```python
from build123d import *

# Parameters (mm, degrees)
CHAMFER1_SIZE      = 0.8
CHAMFER2_SIZE      = 0.5
CUT_EXTRUDE1_DEPTH = 2.5
CHAMFER3_SIZE      = 0.4


with BuildPart() as part:
    # Sketch1 → Revolve1 (revolve)
    with BuildSketch(Plane.XY):
        Polygon((0, 0), (0, 4.25), (5, 4.25), (5, 2.488), (55, 2.488), (55, 0), align=None)
    revolve(axis=Axis((-88.705490849, 0, 0), (1, 0, 0)))

    # Chamfer1
    chamfer1_edges = [part.edges().sort_by_distance(p)[0] for p in [
        (55, -2.488, 0),
    ]]
    chamfer(chamfer1_edges, length=CHAMFER1_SIZE)

    # Chamfer2
    chamfer2_edges = [part.edges().sort_by_distance(p)[0] for p in [
        (0, -4.25, 0),
    ]]
    chamfer(chamfer2_edges, length=CHAMFER2_SIZE)

    # Sketch3 → Cut-Extrude1 (cut)
    with BuildSketch(Plane(origin=(0, 0, 0), x_dir=(0, 0, -1), z_dir=(1, 0, 0))):
        Polygon((-2.309401077, 0), (-1.154700538, -2), (1.154700538, -2), (2.309401077, 0), (1.154700538, 2), (-1.154700538, 2), align=None)
    extrude(amount=CUT_EXTRUDE1_DEPTH, mode=Mode.SUBTRACT)

    # Chamfer3
    chamfer3_edges = [part.edges().sort_by_distance(p)[0] for p in [
        (0, 1, 1.732050808),
        (0, -1, 1.732050808),
        (0, -2, 0),
        (0, -1, -1.732050808),
        (0, 1, -1.732050808),
        (0, 2, 0),
    ]]
    chamfer(chamfer3_edges, length=CHAMFER3_SIZE)


solid = part.part
```
Build history of the part. All positions in model axes, mm. A direction names the side the tool comes from. Give positions to 0.01 mm unless a question says otherwise; leave off trailing zeros. Loops run counter-clockwise (first coordinate to the right, second up) from the corner with the lowest first, then second, coordinate; pieces in that order, holes last. Notation, with made-up numbers: (-12, 66.5) -> (17, 66.5) arc R21 ccw to (17, 72.5) -> close; hole circle Ø5 at (-14.5, 27). An arc over 180 degrees is marked (long way). One line per question, with ' | ' between items. Start each with the question number.
1) 3-axis set-ups, long thin cutter, end or side, ignore diameter. For faces 1 (the cylindrical face through (2.782, 2.285, 3.584)), 2 (the flat face through (0.203, 1.115, 1.893)), 3 (the flat face through (5, 2, -2)): which of +Z, -Z, +X, -X, +Y, -Y reach the whole face in a straight line?
2) Two-plate mould, pull along Z, no slides. Class faces 4 (the flat face through (0, 0.89, -2.45)), 5 (the cylindrical face through (29.944, 2.373, 0.747)), 6 (the flat face through (1, -2, 0)): released by +Z, released by -Z, zero draft, split by the parting line, or undercut.
3) Cut at B-B (x = 44.5). Give the cut face in (y, z), plus the area to 3 significant figures.
4) Probe L1, parallel to X at y = 0.5, z = 2.5; L2, parallel to X at y = -0.5, z = -1; L3, parallel to Y at x = 24, z = -0.25. List the from-to ranges inside material, lowest first.
5) Pin check, flat tips, straight feed: pin 1 (4 mm diameter, centred on x = 29.5, z = 2, fed in from +Y); pin 2 (2 mm diameter, centred on x = 19, y = -1.5, fed in from +Z). Stop position of each tip, or through.
6) Cut at A-A (z = 0). Give the cut face in (x, y), plus the area to 3 significant figures.
Return value:
1) face 1: +X, -X | face 2: -X | face 3: +X
2) face 4: zero draft | face 5: split by the parting line | face 6: undercut
3) outline: circle Ø4.98 at (0, 0) | area: 19.4 mm^2
4) L1: 0 to 5 | L2: 2.5 to 55 | L3: -2.48 to 2.48
5) pin 1: y = 2.49 | pin 2: z = 2.44
6) outline: (0, -3.75) -> (0.5, -4.25) -> (5, -4.25) -> (5, -2.49) -> (54.2, -2.49) -> (55, -1.69) -> (55, 1.69) -> (54.2, 2.49) -> (5, 2.49) -> (5, 4.25) -> (0.5, 4.25) -> (0, 3.75) -> (0, 2.4) -> (0.4, 2) -> (2.5, 2) -> (2.5, -2) -> (0.4, -2) -> (0, -2.4) -> close | area: 280 mm^2
